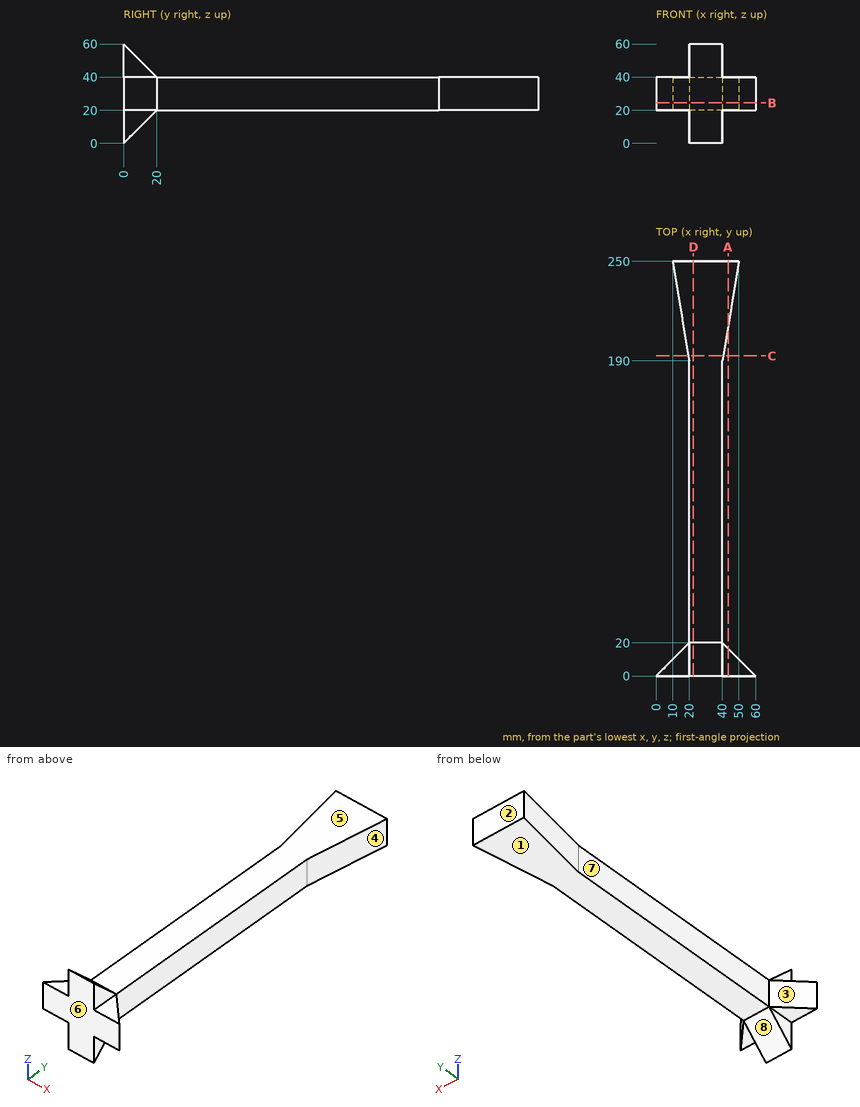
Can you work these out from the drawing? Everything is in mm from the part's minimum corner. A direction names the side the tool comes from. Round coordinates to 2 decimals unless told otherwise and drop trailing zeros. Order: outer loops, then holes, each group sorted by start corner. A loop starts at its lowest first (then second) coordinate and runs counter-clockwise, first axis right, second up. Notation, with made-up numbers: M 3.25,26.25 L 33.25,26.25 A22 ccw 33.25,35.25 Z; hole C -32,-24 d3. An arc over 180 degrees is marked long. Answer as CSV lines item,"result".
Item 1: Imagine slicing it at A-A on x = 43.5. List the corners of the cut face in (y, z) for me, and give its area (3 significant figures).
From the geometry:
outline,"M 0,20 L 16.5,20 L 16.5,40 L 0,40 Z; M 211,20 L 250,20 L 250,40 L 211,40 Z"
area,"1,110 mm2"
Item 2: For pin 1 (4 mm diameter, centred on x = 37.5, y = 97.5, fed in from +Z); pin 2 (6 mm diameter, centred on y = 87, z = 27.5, fed in from -X); pin 3 (12 mm diameter, centred on y = 224, z = 22.5, fed in from -X), each with a flat end and sliding along its axis, tell me the tip position at first contact or that it passes through.
From the geometry:
pin 1,"z = 40"
pin 2,"x = 20"
pin 3,"x = 13.33"
Item 3: Imagine slicing it at C-C on y = 193. List the corners of the cut face in (x, z) for me.
From the geometry:
outline,"M 19.5,20 L 40.5,20 L 40.5,40 L 19.5,40 Z"
Item 4: Imagine slicing it at B-B on z = 24.5. List the corners of the cut face in (x, y) for me, and give its area (3 significant figures).
From the geometry:
outline,"M 0,0 L 60,0 L 40,20 L 40,190 L 50,250 L 10,250 L 20,190 L 20,20 Z"
area,"6,000 mm2"
Item 5: Imagine slicing it at D-D on x = 22.5. List the corners of the cut face in (y, z) for me, and give its area (3 significant figures).
From the geometry:
outline,"M 0,0 L 20,20 L 250,20 L 250,40 L 20,40 L 0,60 Z"
area,"5,400 mm2"
Item 6: Which directions (+Z, -Z, +X, -X, +Y, -Y) give clear straight access to the entire face, cutting with the end or side of a thin tool? Please do the marked faces 4, 5, 6, 7 and 8.
From the geometry:
face 4,"+Z, -Z, +X"
face 5,"+Z, +X, -X, +Y"
face 6,"+Z, -Z, +X, -X, -Y"
face 7,"+Z, -Z, -X"
face 8,"-Z, +X, -X, +Y"
Item 7: Please list where these lines run through material, in increasing order: L1, parallel to X at y = 83, z = 32.5; L2, parallel to Y at x = 37, z = 16. Write a range as [from, to].
From the geometry:
L1,"[20, 40]"
L2,"[0, 16]"
Item 8: We'd pull the mould along Y, two halves only. Please class the marked faces 1, 2 and 3: +Y half, -Y half, draft (parallel to the pull), parting line (faces both ways), or undercut.
From the geometry:
face 1,"draft"
face 2,"+Y half"
face 3,"undercut"
